Can you work these out from the drawing? Everything is in mm from the part's minimum corner. Coordinates: 2 decimals unless noted, no trailing zeros. Order: outer loops, then holes, each group sorted by start corner. A loop starts at its lowest first (then second) coordinate and runs counter-clockwise, first axis right, second up. Notation, with made-up numbers: (22.5, 66.25) - (68.5, 66.25) arc R13 cw to (68.5, 84.25) - close; hole circle Ø5 at (-32, -7). An arc over 180 degrees is marked (long way). Use a Markdown table: item, result. Add a question column.
(1) I want a section at D-D (x = 19.5). List the corners of the cut face in (y, z) for me.
(2) I want a section at B-B (z = 61). List the corners of the cut face in (x, y) for me.
(3) I want a section at C-C (y = 2.85). State how many separate pieces and enclosed holes the cut face has, and give its area (3 significant figures).
(4) If I drill on L1, parallel to Z at x = 107, y = 3.15; L2, parallel to Z at x = 140.5, y = 2.4 (1 decimal); L3, parallel to X at y = 2.3, z = 76.5, over which ranges is the centre line in solid material (lowest first)? Write a range as [from, to].
(5) For pin 1 Ø3 at (x, y) = (213.5, 4.5) entering from +Z (1 decimal); pin 2 Ø2 at (x, y) = (82.5, 4.5) entering from +Z; pin 3 Ø2 at (x, y) = (185, 2) entering from -Z, each with a flat end and sliding along its axis, tell me the tip position at first contact or that it passes through.
(6) I want a section at A-A (x = 125). List the corners of the cut face in (y, z) for me.
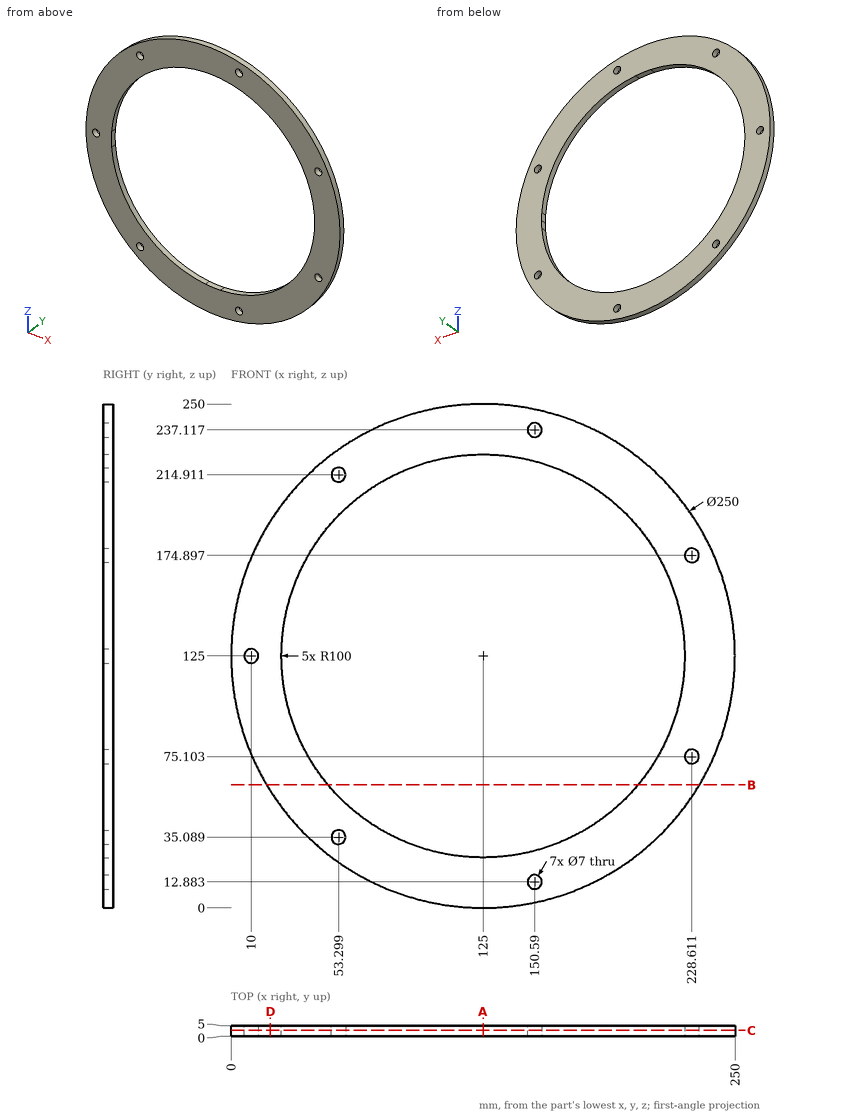
Answers follow:
| question | item | result |
|---|---|---|
| 1 | outline | (0, 57.96) - (5, 57.96) - (5, 192.04) - (0, 192.04) - close |
| 2 | outline | (17.63, 0) - (48.16, 0) - (48.16, 5) - (17.63, 5) - close; (201.84, 0) - (232.37, 0) - (232.37, 5) - (201.84, 5) - close |
| 3 | separate pieces | 1 |
| 3 | enclosed holes | 8 |
| 3 | area | 17,400 mm² |
| 4 | L1 | z = [1.3, 26.63], [223.37, 248.7] |
| 4 | L2 | z = [1, 26.2], [223.8, 249] |
| 4 | L3 | x = [9.79, 37.55], [212.45, 225.4], [231.82, 240.21] |
| 5 | pin 1 | stops at z = 214.8 |
| 5 | pin 2 | stops at z = 242.91 |
| 5 | pin 3 | stops at z = 14.8 |
| 6 | outline | (0, 0) - (5, 0) - (5, 25) - (0, 25) - close; (0, 225) - (5, 225) - (5, 250) - (0, 250) - close |
